Geometry: see drawing. Coordinates: mm, zero at the bounding-box minimum. Coordinates: 2 decimals unless noted, no trailing zeros. Loops run counter-clockwise (first coordinate to the right, second up) from the corner with the lowest first, then second, coordinate; pieces in that order, holes last. Notation, with made-up numbers: (-19.5, 6.25) -> (-2.5, 6.25) arc R15 ccw to (-2.5, 10.25) -> close; hole circle Ø10 at (-20, 40). An arc over 180 degrees is marked (long way). Answer as a JSON object with one key per item and string values.
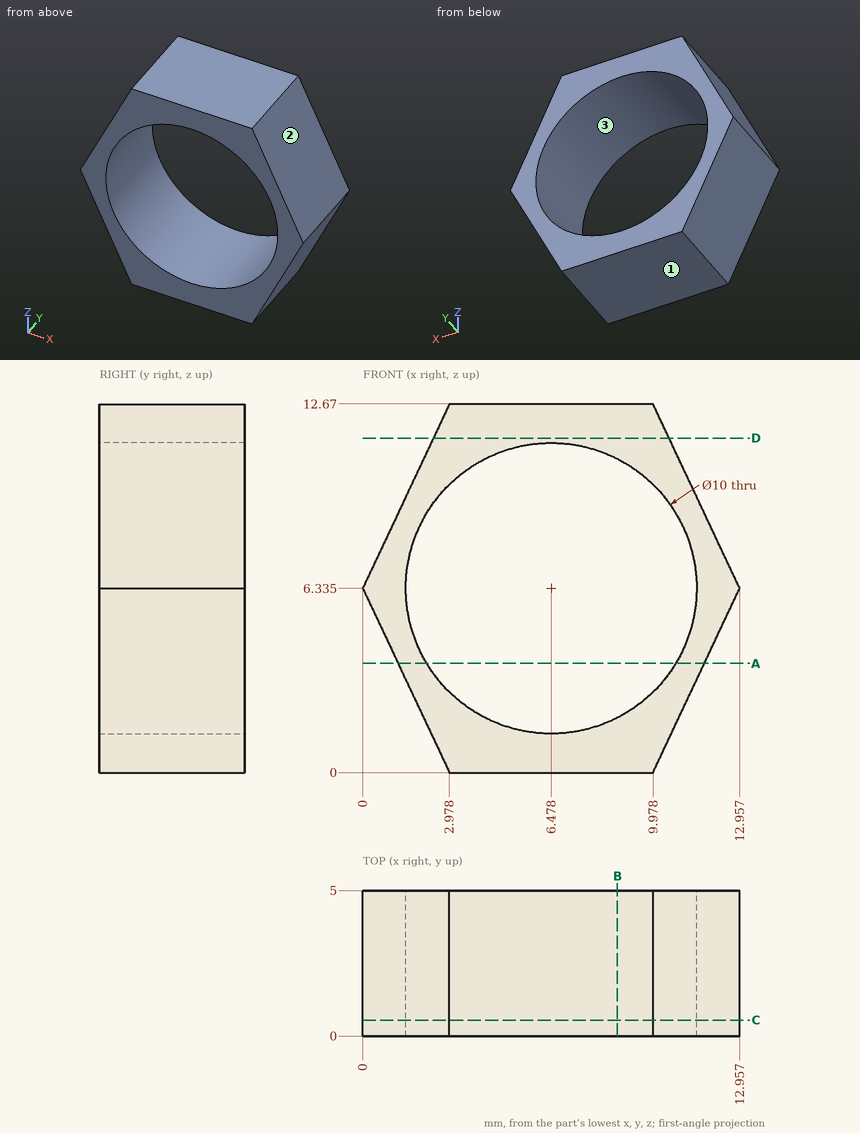
1. Mould query, pull axis X, two halves, no side actions, for the marked faces 1, 2 and 3. Classes: pulls with the +X half, pulls with the -X half, needs draft (parallel to the pull), parting line crosses it, or undercut.
Reply:
{"face 1": "needs draft", "face 2": "pulls with the +X half", "face 3": "undercut"}
2. Section query C-C (y = 0.55). Return loops of the section in (x, z) (1 decimal).
Reply:
{"outline": "(0, 6.3) -> (3, 0) -> (10, 0) -> (13, 6.3) -> (10, 12.7) -> (3, 12.7) -> close; hole circle Ø10 at (6.5, 6.3)"}
3. Section query D-D (z = 11.5). Return loops of the section in (x, y).
Reply:
{"outline": "(2.43, 0) -> (10.53, 0) -> (10.53, 5) -> (2.43, 5) -> close"}
4. Pin query (flat end, axial travel): P1, Ø2, axis at y = 3, z = 8, coming from the +X side. Return the tip coordinate at first contact, or that it passes through.
Reply:
{"P1": "stops at x = 12.64"}
5. Line query: line 1 along Z through (x, y) = (7.75, 0.9); line 2 along X through (y, z) = (1.75, 6); line 3 along Z through (x, y) = (9.5, 4.4). Output: solid intervals per line, ascending.
Reply:
{"line 1": "z = 0 to 1.5, 11.17 to 12.67", "line 2": "x = 0.16 to 1.49, 11.47 to 12.8", "line 3": "z = 0 to 2.35, 10.32 to 12.67"}
6. Section query B-B (x = 8.75). Return loops of the section in (y, z).
Reply:
{"outline": "(0, 0) -> (5, 0) -> (5, 1.88) -> (0, 1.88) -> close; (0, 10.79) -> (5, 10.79) -> (5, 12.67) -> (0, 12.67) -> close"}
7. Section query A-A (z = 3.75). Return loops of the section in (x, y) (1 decimal).
Reply:
{"outline": "(1.2, 0) -> (2.2, 0) -> (2.2, 5) -> (1.2, 5) -> close; (10.8, 0) -> (11.7, 0) -> (11.7, 5) -> (10.8, 5) -> close"}
